Design review of the part built by this model. Coordinates are the model's own, in mm. A direction names the side the tool comes from. Round coordinates to 2 decimals unless told otherwise and drop trailing zeros. Write each loop counter-clockwise with the first axis right and the second up, starting at its lowest first coordinate (ties: lowest second). Pieces come first, ordered by that corner, then holes. Notation, with made-up numbers: (26.5, 74.25) -> (33.5, 74.25) arc R28 cw to (33.5, 101.25) -> close; hole circle Ø8 at (54.5, 13). An arc over 180 degrees is marked (long way). Write item = value, one per line. Start each with the question number.
Item 1: To check wall thickness, follow L1, parallel to Z at x = 5, y = -16.5; L2, parallel to X at y = 23.5, z = 47.5; L3, parallel to X at y = -16.5, z = 63. State the ranges of each line that lie inside material, in increasing order.
Item 2: For pin 1 Ø3 at (y, z) = (28.5, 49) entering from +X; pin 2 Ø4 at (y, z) = (-25.5, 37.5) entering from +X; pin 3 Ø3 at (x, z) = (25.5, 5.5) entering from +Y, all flat-tipped, find the tip position at first contact; note any pin that passes through.
Item 3: Mouldability with a two-part tool opening along Z and no side actions: class faces 6 (the conical face through (-4.729, -21.294, -0.516)), 7 (the flat face through (-0.1, 21.5, 76.503)), 8 (the conical face through (27.02, -11.2, 71.97)), 9 (the cylindrical face through (-16.94, -12.99, 74.47)) as released by +Z, released by -Z, zero draft, split by the parting line, or undercut.
Item 4: Add section A-A, the plane z = 5. State the section outline as (x, y) points.
Item 5: Machinability: for faces 1 (the flat face through (-15, 25, -8.254)), 2 (the flat face through (0, 0, 0)), 3 (the cylindrical face through (21.385, 33.541, 31.564)), 4 (the flat face through (0.1, 21.5, 72.497)), 5 (the flat face through (0, 0, 3.542)), which of the approach directions +Z, -Z, +X, -X, +Y, -Y give a long, thin tool a straight path to every point of the face, cutting with its end or side? Answer none if there is none.
from build123d import *


with BuildPart() as f1:
    # F0 (on Front) → F1 (revolve)
    with BuildSketch(Plane.XZ):
        with BuildLine():
            Line((0, 3.541697), (0, 0))
            Line((0, 0), (21.348186, 0))
            Line((21.348186, 0), (28.781075, -8.254268))
            Line((28.781075, -8.254268), (33.428356, -8.254268))
            ThreePointArc((33.428356, -8.254268), (37.918484, -6.394396), (39.778356, -1.904268))
            Line((39.778356, -1.904268), (39.778356, 64.10753))
            Line((39.778356, 64.10753), (28.781075, 76.502554))
            Line((28.781075, 76.502554), (21.348186, 76.502554))
            Line((21.348186, 76.502554), (21.348186, 72.496518))
            Line((21.348186, 72.496518), (28.781075, 72.496518))
            Line((28.781075, 72.496518), (36.224067, 64.10753))
            Line((36.224067, 64.10753), (36.224067, -4.835905))
            Line((36.224067, -4.835905), (28.781075, -4.835905))
            Line((28.781075, -4.835905), (24.490498, 0))
            Line((24.490498, 0), (21.348186, 3.541697))
            Line((21.348186, 3.541697), (0, 3.541697))
        make_face()
    revolve(axis=Axis((0, 0, 34.186214), (0, 0, 1)))


solid = f1.part
Result set:
q1.L1 = 0 to 3.54
q1.L2 = -32.09 to -27.57, 27.57 to 32.09
q1.L3 = -36.19 to -32.25, 32.25 to 36.19
q2.pin_1 = 29.21
q2.pin_2 = 32.09
q2.pin_3 = 31.72
q3.face_6 = released by -Z
q3.face_7 = released by +Z
q3.face_8 = undercut
q3.face_9 = zero draft
q4.outline = circle Ø79.56 at (0, 0); hole circle Ø72.45 at (0, 0)
q5.face_1 = -Z, +X, -X, +Y, -Y
q5.face_2 = -Z
q5.face_3 = +Z, -Z
q5.face_4 = none
q5.face_5 = +Z
